```python
from build123d import *

# Parameters (mm, degrees)
SKETCH1_W         = 1816.1
SKETCH1_H         = 774.7
BASE_DEPTH        = 6.35
SKETCH2_W         = 15.875
SKETCH2_H         = 50.8
RIB_RELIEF_DEPTH  = 1194.631105074
CUTOUT_DEPTH      = 1194.631105074
CUTOUT_DEPTH_BACK = 1194.631105074


with BuildPart() as part:
    # Sketch1 → base (new body)
    with BuildSketch(Plane.XY):
        with Locations((0, 387.35)):
            Rectangle(SKETCH1_W, SKETCH1_H)
    extrude(amount=BASE_DEPTH)

    # Sketch2 → rib-relief (cut, through all)
    with BuildSketch(Plane.XY.offset(6.35)):
        with Locations((-300.0375, 749.3)):
            Rectangle(SKETCH2_W, SKETCH2_H)
        with Locations((300.0375, 749.3)):
            Rectangle(SKETCH2_W, SKETCH2_H)
    extrude(amount=-RIB_RELIEF_DEPTH, mode=Mode.SUBTRACT)

    # Sketch3 → cutout (cut, two sides: drawn at the far end of the back side and taken through both)
    with BuildSketch(Plane.XY.offset(6.35).offset(-CUTOUT_DEPTH_BACK)):
        with BuildLine():
            Line((-40, 720.725), (40, 720.725))
            ThreePointArc((40, 720.725), (76.825, 683.9), (40, 647.075))
            Line((40, 647.075), (-40, 647.075))
            ThreePointArc((-40, 647.075), (-76.825, 683.9), (-40, 720.725))
        make_face()
    extrude(amount=CUTOUT_DEPTH + CUTOUT_DEPTH_BACK, mode=Mode.SUBTRACT)


solid = part.part
```
Check sheet for the modelled part. Datum: model origin and axes. Units: mm. Round coordinates to 2 decimals unless told otherwise and drop trailing zeros. Loops run counter-clockwise (first coordinate to the right, second up) from the corner with the lowest first, then second, coordinate; pieces in that order, holes last. Notation, with made-up numbers: (23, 48.5) - (34, 48.5) arc R25 cw to (34, 81.5) - close; hole circle Ø3 at (-16, 85). An arc over 180 degrees is marked (long way). Answer as a JSON object with one key per item and string values. Group by question number.
Q1. Mould release check, pull along X, two halves, no side actions. Record for faces 1 (the face through (-76.816, 683.09, 3.131)), 2 (the face through (76.816, 684.71, 3.131)), 3 (the face through (-13, 393, 6.35)): released by +X, released by -X, zero draft, split by the parting line, or undercut.
Q2. Scan lines: line 1 along Y through (x, z) = (-6.5, 3.25) (3 decimals); line 2 along Y through (x, z) = (-73, 2); line 3 along X through (y, z) = (669.5, 4.25). Record each from-to range of solid material in increasing order. Write a range as [from, to].
Q3. Sectioned sample at A-A, the plane y = 683.9. Enter the section's corners in (x, z) (3 decimals).
Q4. Gauge pin test, flat end, axial feed: P1, Ø3, axis at x = 298, z = 4.5, coming from the +Y side. Record the tip position at first contact, or that the pin passes through.
Solution:
{
 "1": {"face 1": "undercut", "face 2": "undercut", "face 3": "zero draft"},
 "2": {"line 1": "y = [0, 647.075], [720.725, 774.7]", "line 2": "y = [0, 667.56], [700.24, 774.7]", "line 3": "x = [-908.05, -73.89], [73.89, 908.05]"},
 "3": {"outline": "(-908.05, 0) - (-76.825, 0) - (-76.825, 6.35) - (-908.05, 6.35) - close; (76.825, 0) - (908.05, 0) - (908.05, 6.35) - (76.825, 6.35) - close"},
 "4": {"P1": "stops at y = 723.9"}
}
